Can you work these out from the drawing? Everything is in mm from the part's minimum corner. Coordinates: 2 decimals unless noted, no trailing zeros. Order: outer loops, then holes, each group sorted by start corner. A loop starts at its lowest first (then second) coordinate and runs counter-clockwise, first axis right, second up. Notation, with made-up numbers: (86.25, 71.25) -> (104.25, 71.25) arc R18 cw to (104.25, 84.25) -> close; hole circle Ø6 at (63, 49.5). An arc over 180 degrees is marked (long way). Put each result on its own line as item: value. Start each with the question number.
Q1. Will this pin go through, and if not, where does the flat tip stop? pin 1 (3 mm diameter, centred on x = 30.07, z = 37.5, fed in from -Y) (3 decimals).
Q2. If we section it at A-A (z = 37.5): Please give me the cut outline in (x, y).
Q3. Please list where these lines run through material, in increasing order: line 1 along X through (y, z) = (7.5, 37.5); line 2 along Z through (x, y) = (30, 1.25); line 3 along Z through (x, y) = (31, 8.5).
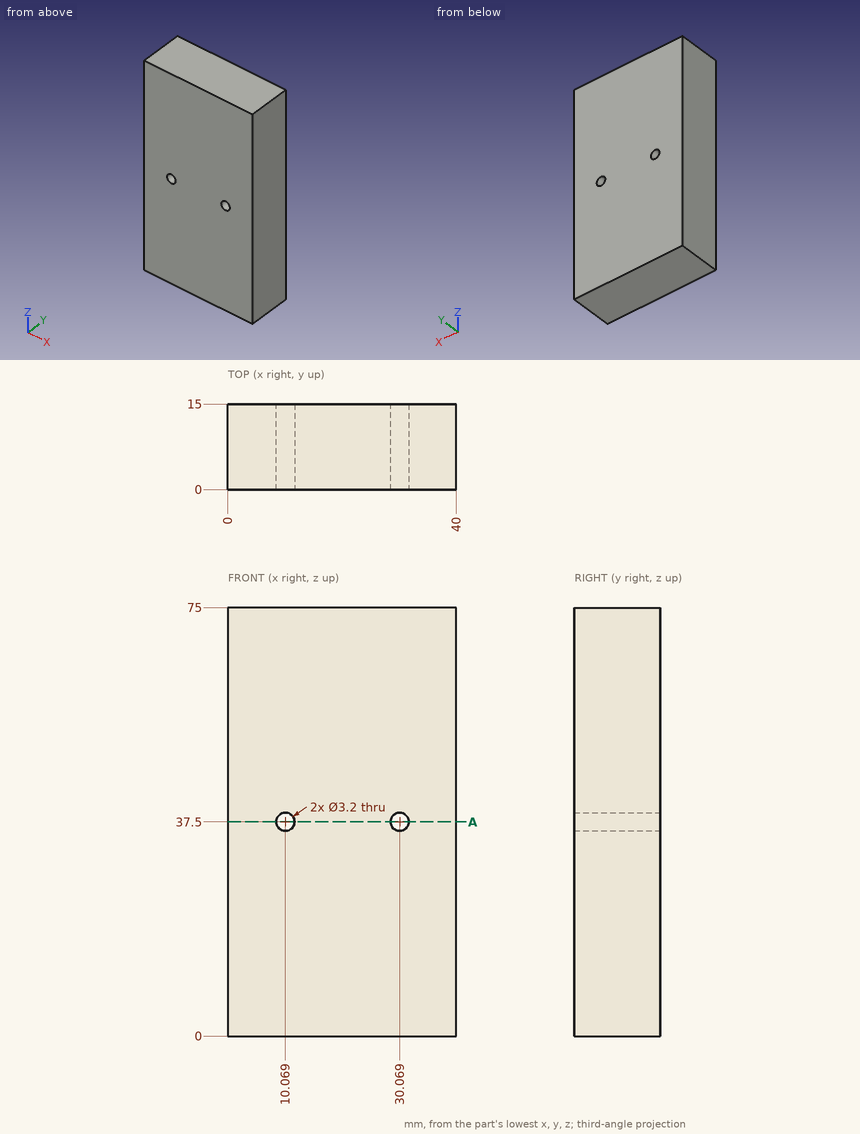
The answers:
1. pin 1: through
2. outline: (0, 0) -> (8.47, 0) -> (8.47, 15) -> (0, 15) -> close; (11.67, 0) -> (28.47, 0) -> (28.47, 15) -> (11.67, 15) -> close; (31.67, 0) -> (40, 0) -> (40, 15) -> (31.67, 15) -> close
3. line 1: 0 to 8.47, 11.67 to 28.47, 31.67 to 40
3. line 2: 0 to 35.9, 39.1 to 75
3. line 3: 0 to 36.2, 38.8 to 75
